Autodesk Inventor part; units mm, degrees
ref_plane "YZ Plane" through (0, 0, 0) normal (1, 0, 0) x (0, 1, 0)
ref_plane "XZ Plane" through (0, 0, 0) normal (0, 1, 0) x (-1, 0, 0)
ref_plane "XY Plane" through (0, 0, 0) normal (0, 0, 1) x (1, 0, 0)
sketch "Sketch1" plane through (0, 0, 0) normal (0, 1, 0) x (-1, 0, 0)
  circle A0 centre (0, 0) radius 190.5
  dimension "d1" = 381
ref_plane "Work Plane1" through (0, 12.7, 0) normal (0, 1, 0) x (1, 0, 0)
sketch "Sketch2" plane through (0, 12.7, 0) normal (0, 1, 0) x (1, 0, 0)
  line L0 (0, 0) -> (0, -177.8) construction
  line L1 (0, 0) -> (177.8, 0) construction
  circle A0 centre (0, -177.8) radius 3.81
  circle A1 centre (153.9793, -88.9) radius 3.81
  circle A2 centre (153.9793, 88.9) radius 3.81
  circle A3 centre (0, 177.8) radius 3.81
  circle A4 centre (-153.9793, 88.9) radius 3.81
  circle A5 centre (-153.9793, -88.9) radius 3.81
  dimension "d6" = 177.8
  dimension "d7" = 90
  dimension "d8" = 7.62
  dimension "d9" = 360
extrude "Extrusion3" add sketch "Sketch1" along normal blind 12.7
extrude "Extrusion4" cut sketch "Sketch2" against normal through all
sketch "Sketch3" plane through (0, 0, 0) normal (0, -1, 0) x (1, 0, 0)
  circle A0 centre (0, 0) radius 162.56
  dimension "d16" = 325.12
extrude "Extrusion5" cut sketch "Sketch3" against normal blind 9.8806
fillet "Fillet1" radius 3.175 1 edges at (190.5, 12.7, 0)
sketch "Sketch4" plane through (0, 12.7, 0) normal (0, 1, 0) x (1, 0, 0)
  arc A0 (-12.6214, -55.7389) -> (12.6214, -55.7389) centre (0, 0) ccw
  arc A1 (-12.6214, -55.7389) -> (12.6214, -55.7389) centre (0, -57.15) ccw
  dimension "d20" = 114.3
  dimension "d21" = 25.4
extrude "Extrusion6" cut sketch "Sketch4" against normal blind 9.8806
properties part number "Turntable Cap" material "PVC-Piping"
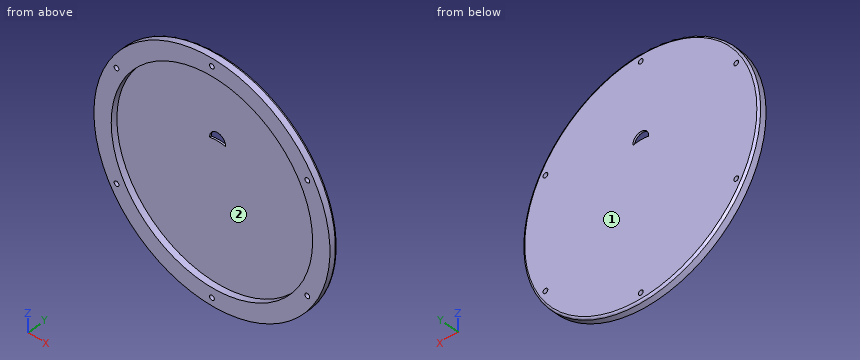
The listing builds one solid part. Answer for the finished solid, in the listing's coordinates (mm). Face numbers are marked on the shaded views. Coordinates: 2 decimals unless noted, no trailing zeros. Loops run counter-clockwise (first coordinate to the right, second up) from the corner with the lowest first, then second, coordinate; pieces in that order, holes last. Notation, with made-up numbers: (-8.75, 24.25) -> (19.25, 24.25) arc R19 ccw to (19.25, 50.25) -> close; hole circle Ø10 at (-31.75, -32.75). An arc over 180 degrees is marked (long way). Write item = value, one per line. Start each with the question number.
1) Straight lines are drawn through the part: line 1 (Z direction, x = 0, y = 5.5); line 2 (Z direction, x = 0, y = 10.25); line 3 (Y direction, x = -153, z = 8.5). For each, find the intervals that lie inside material, in ascending order. Write a range as from..to.
2) Given pin 1 Ø1.5 at (x, y) = (-61, 7) entering from +Z; pin 2 Ø2 at (x, y) = (147, 8.5) entering from -Z; pin 3 Ø4 at (x, y) = (-64, 3.5) entering from +Z, each flat-ended and moving along its own axis, determine where each tip first touches the part or whether it passes through.
3) A cutting plane is placed at A-A (z = 0). Give the vertices of the cut face in (x, y) (3 decimals), then the cut area to 3 significant figures.
4) The mould has two halves that part along X. Classify the marked faces 1 and 2: released by +X, released by -X, zero draft, split by the parting line, or undercut.
Responses:
q1.line_1 = -190.5..-181.61, -173.99..-162.56, 162.56..173.99, 181.61..190.5
q1.line_2 = -190.42..-181.61, -173.99..57.15, 69.85..173.99, 181.61..190.42
q1.line_3 = 9.88..12.7
q2.pin_1 = 180.72
q2.pin_2 = -122.37
q2.pin_3 = 180.13
q3.outline = (-190.5, 0) -> (-162.56, 0) -> (-162.56, 9.881) -> (162.56, 9.881) -> (162.56, 0) -> (190.5, 0) -> (190.5, 9.525) arc R3.175 ccw to (187.325, 12.7) -> (-187.325, 12.7) arc R3.175 ccw to (-190.5, 9.525) -> close
q3.area = 1,620 mm²
q4.face_1 = zero draft
q4.face_2 = undercut
